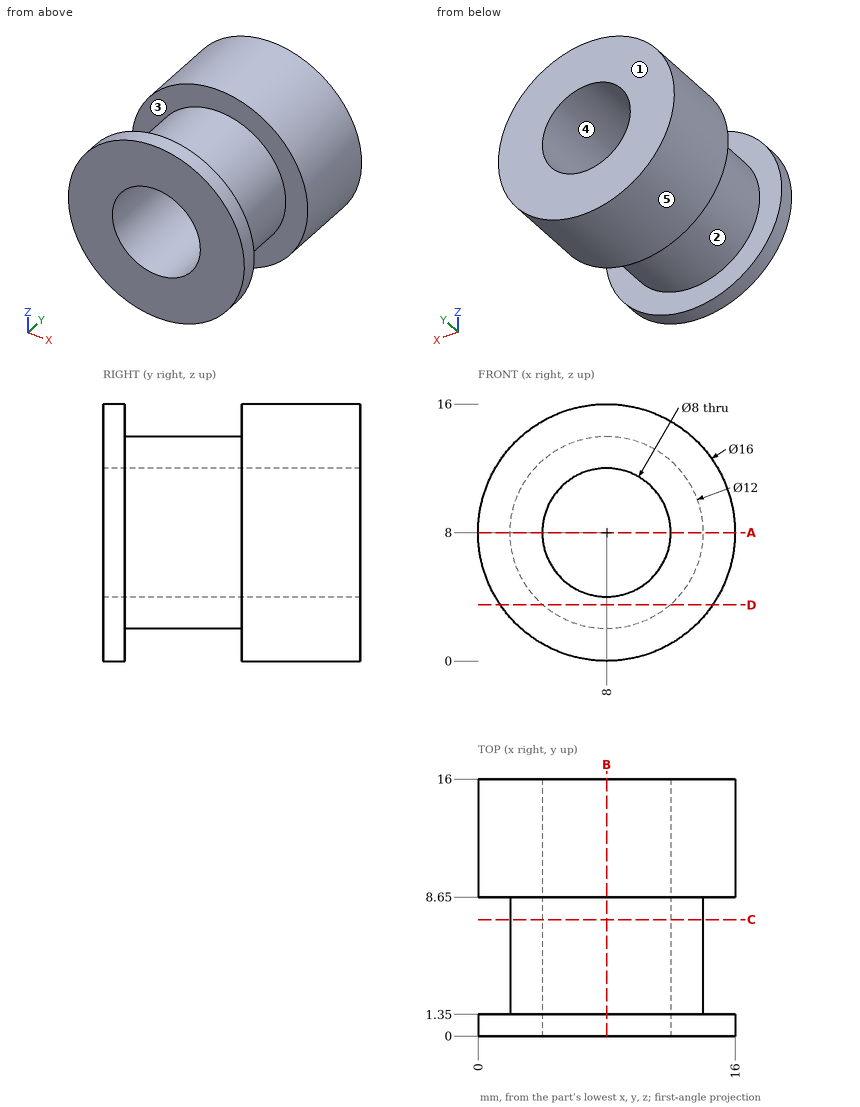
Input: dimensioned drawing with shaded views. Units: mm. Origin: part minimum x, y, z. A direction names the side the tool comes from. Round coordinates to 2 decimals unless told otherwise and drop trailing zeros. Loops run counter-clockwise (first coordinate to the right, second up) from the corner with the lowest first, then second, coordinate; pieces in that order, holes last. Notation, with made-up numbers: M 61.25,40 L 118.25,40 A27 cw 118.25,66 Z; hole C 55.25,-29 d4. An arc over 180 degrees is marked long. Return JSON: item names as keys, results as strings. Group by question number.
1. Material intervals for line 1 along Y through (x, z) = (14.75, 11); line 2 along X through (y, z) = (11.5, 8); line 3 along X through (y, z) = (6.75, 8), sorted ascending. Write a range as from..to.
2. Section query B-B on x = 8. Output: boundary loops of the cut face in (y, z).
3. Section query D-D on z = 3.5. Output: boundary loops of the cut face in (x, y), and give its area (3 significant figures).
4. Section query A-A on z = 8. Output: boundary loops of the cut face in (x, y), and give its area (3 significant figures).
5. Reachability of the marked faces 1 and 2 from +Z, -Z, +X, -X, +Y, -Y: full face, straight path, thin tool, end or side. Return the list, or none.
6. Section query C-C on y = 7.25. Output: boundary loops of the cut face in (x, z), and give its area (3 significant figures).
7. Pin query (flat end, axial travel): pin 1 (5 mm diameter, centred on x = 6.5, z = 4.5, fed in from -Y); pin 2 (3 mm diameter, centred on x = 12, y = 9.5, fed in from +Z); pin 3 (1 mm diameter, centred on x = 5.5, y = 3.5, fed in from -Z). Return the tip coordinate at first contact, or that it passes through.
8. Mould query, pull axis X, two halves, no side actions, for the marked faces 3, 4 and 5. Classes: released by +X, released by -X, zero draft, split by the parting line, or undercut.
Checks:
{
 "1": {"line 1": "y = 0..1.35, 8.65..16", "line 2": "x = 0..4, 12..16", "line 3": "x = 2..4, 12..14"},
 "2": {"outline": "M 0,0 L 1.35,0 L 1.35,2 L 8.65,2 L 8.65,0 L 16,0 L 16,4 L 0,4 Z; M 0,12 L 16,12 L 16,16 L 8.65,16 L 8.65,14 L 1.35,14 L 1.35,16 L 0,16 Z"},
 "3": {"outline": "M 1.39,0 L 14.61,0 L 14.61,1.35 L 11.97,1.35 L 11.97,8.65 L 14.61,8.65 L 14.61,16 L 1.39,16 L 1.39,8.65 L 4.03,8.65 L 4.03,1.35 L 1.39,1.35 Z", "area": "173 mm²"},
 "4": {"outline": "M 0,0 L 4,0 L 4,16 L 0,16 L 0,8.65 L 2,8.65 L 2,1.35 L 0,1.35 Z; M 12,0 L 16,0 L 16,1.35 L 14,1.35 L 14,8.65 L 16,8.65 L 16,16 L 12,16 Z", "area": "98.8 mm²"},
 "5": {"face 1": "+Z, -Z, +X, -X, +Y", "face 2": "none"},
 "6": {"outline": "C 8,8 d12; hole C 8,8 d8", "area": "62.8 mm²"},
 "7": {"pin 1": "stops at y = 0", "pin 2": "stops at z = 15.6", "pin 3": "stops at z = 2.34"},
 "8": {"face 3": "zero draft", "face 4": "undercut", "face 5": "split by the parting line"}
}
